from build123d import *

# Parameters (mm, degrees)
SKETCH2_R                = 107.15
BOSS_EXTRUDE2_DEPTH      = 70
BOSS_EXTRUDE2_DEPTH_BACK = 70
SKETCH10_R               = 19
CUT_EXTRUDE2_DEPTH       = 10
SKETCH18_R               = 22.5
BOSS_EXTRUDE6_DEPTH      = 32
BOSS_EXTRUDE6_DEPTH_BACK = 1
SKETCH56_R               = 30.95
BOSS_EXTRUDE7_DEPTH      = 5
BOSS_EXTRUDE7_DEPTH_BACK = 6
SKETCH20_R               = 104.1
CUT_EXTRUDE3_DEPTH       = 140
SKETCH51_R               = 2.5
CUT_EXTRUDE14_DEPTH      = 5
CUT_EXTRUDE14_DEPTH_BACK = 55
CUT_EXTRUDE15_DEPTH      = 5
SKETCH44_R               = 7.5
CUT_EXTRUDE10_DEPTH      = 10
FILLET3_R                = 1.5
SKETCH61_R               = 104.15
BOSS_EXTRUDE8_DEPTH      = 2
SKETCH62_R               = 102.15
CUT_EXTRUDE16_DEPTH      = 10
CHAMFER7_SIZE            = 1
CHAMFER7_SIZE2           = 0.700207538
SKETCH5_W                = 211.3
SKETCH5_H                = 3
BOSS_EXTRUDE3_DEPTH      = 24
SKETCH24_R               = 18.25
CUT_EXTRUDE6_DEPTH       = 50
SKETCH23_R               = 20.45
CUT_EXTRUDE5_DEPTH       = 7
CUT_EXTRUDE5_DEPTH_BACK  = 5
CHAMFER1_SIZE            = 0.5
FILLET4_R                = 0.6
CUT_EXTRUDE19_DEPTH      = 4


with BuildPart() as part:
    # Sketch2 → Boss-Extrude2 (new, two sides)
    with BuildSketch(Plane.XY) as boss_extrude2_sk:
        Circle(SKETCH2_R)
    extrude(amount=BOSS_EXTRUDE2_DEPTH)
    extrude(boss_extrude2_sk.sketch, amount=-BOSS_EXTRUDE2_DEPTH_BACK)

    # Sketch10 → Cut-Extrude2 (cut, symmetric)
    with BuildSketch(Plane(origin=(0, 51.109455148, -37.133192748), x_dir=(1, 0, 0), z_dir=(0, -0.8090169943749408, 0.5877852522924822))):
        with Locations((0, 95.341869558)):
            Circle(SKETCH10_R)
    extrude(amount=CUT_EXTRUDE2_DEPTH, both=True, mode=Mode.SUBTRACT)

    # Sketch18 → Boss-Extrude6 (add, two sides)
    with BuildSketch(Plane(origin=(0, 63.244710063, -45.949971532), x_dir=(1, 0, 0), z_dir=(0, -0.8090169943749408, 0.5877852522924822))) as boss_extrude6_sk:
        with Locations((0, 95.341869558)):
            Circle(SKETCH18_R)
    extrude(amount=BOSS_EXTRUDE6_DEPTH)
    extrude(boss_extrude6_sk.sketch, amount=-BOSS_EXTRUDE6_DEPTH_BACK)

    # Sketch56 → Boss-Extrude7 (add, two sides)
    with BuildSketch(Plane(origin=(0, -107.15, 0), x_dir=(1, 0, 0), z_dir=(0, 1, 0))) as boss_extrude7_sk:
        with Locations(Location((0, 1.5, 0), (0, 0, 270))):
            Circle(SKETCH56_R)
    extrude(amount=BOSS_EXTRUDE7_DEPTH)
    extrude(boss_extrude7_sk.sketch, amount=-BOSS_EXTRUDE7_DEPTH_BACK)

    # Sketch20 → Cut-Extrude3 (cut)
    with BuildSketch(Plane.XY.offset(70)):
        Circle(SKETCH20_R)
    extrude(amount=-CUT_EXTRUDE3_DEPTH, mode=Mode.SUBTRACT)

    # Sketch51 → Cut-Extrude14 (cut, two sides)
    with BuildSketch(Plane(origin=(0, -107.15, 0), x_dir=(1, 0, 0), z_dir=(0, 1, 0))) as cut_extrude14_sk:
        with Locations(Location((0, -24, 0), (0, 0, 90))):
            Circle(SKETCH51_R)
    extrude(amount=CUT_EXTRUDE14_DEPTH, mode=Mode.SUBTRACT)
    extrude(cut_extrude14_sk.sketch, amount=-CUT_EXTRUDE14_DEPTH_BACK, mode=Mode.SUBTRACT)

    # Sketch58 → Cut-Extrude15 (cut)
    with BuildSketch(Plane(origin=(0, -105.15, 0), x_dir=(1, 0, 0), z_dir=(0, 1, 0))):
        Polygon((0, -24), (1, -24), (1, -34.192827208), (-1, -34.192827208), (-1, -24), align=None)
    extrude(amount=CUT_EXTRUDE15_DEPTH, mode=Mode.SUBTRACT)

    # Sketch44 → Cut-Extrude10 (cut)
    with BuildSketch(Plane(origin=(0, -105.15, 0), x_dir=(1, 0, 0), z_dir=(0, 1, 0))):
        with Locations((0, -35.5)):
            Circle(SKETCH44_R)
    extrude(amount=CUT_EXTRUDE10_DEPTH, mode=Mode.SUBTRACT)

    # Fillet3
    fillet3_edges = [part.edges().sort_by_distance(p)[0] for p in [
        (0, -105.15, 26.5),
    ]]
    fillet(fillet3_edges, radius=FILLET3_R)

    # Sketch61 → Boss-Extrude8 (add)
    with BuildSketch(Plane.XY.offset(22)):
        Circle(SKETCH61_R)
    extrude(amount=-BOSS_EXTRUDE8_DEPTH)

    # Sketch62 → Cut-Extrude16 (cut)
    with BuildSketch(Plane.XY.offset(22)):
        Circle(SKETCH62_R)
    extrude(amount=-CUT_EXTRUDE16_DEPTH, mode=Mode.SUBTRACT)

    # Chamfer7
    chamfer7_edges = [part.edges().sort_by_distance(p)[0] for p in [
        (-102.15, 0, 20),
    ]]
    chamfer7_side = [part.faces().sort_by_distance(p)[0] for p in [
        (-102.15, 0, 21),
    ]]
    chamfer(chamfer7_edges, length=CHAMFER7_SIZE, length2=CHAMFER7_SIZE2, reference=chamfer7_side[0])

    # Sketch5 → Boss-Extrude3 (add)
    with BuildSketch(Plane.XY.offset(45)):
        Rectangle(SKETCH5_W, SKETCH5_H)
    extrude(amount=-BOSS_EXTRUDE3_DEPTH)

    # Sketch24 → Cut-Extrude6 (cut)
    with BuildSketch(Plane(origin=(0, 63.244710063, -45.949971532), x_dir=(1, 0, 0), z_dir=(0, -0.8090169943749408, 0.5877852522924822))):
        with Locations(Location((0, 95.341869558, 0), (0, 0, 244.88549582))):
            Circle(SKETCH24_R)
    extrude(amount=CUT_EXTRUDE6_DEPTH, mode=Mode.SUBTRACT)

    # Sketch23 → Cut-Extrude5 (cut, two sides)
    with BuildSketch(Plane(origin=(0, 63.244710063, -45.949971532), x_dir=(1, 0, 0), z_dir=(0, -0.8090169943749408, 0.5877852522924822))) as cut_extrude5_sk:
        with Locations(Location((0, 95.341869558, 0), (0, 0, 270))):
            Circle(SKETCH23_R)
    extrude(amount=CUT_EXTRUDE5_DEPTH, mode=Mode.SUBTRACT)
    extrude(cut_extrude5_sk.sketch, amount=-CUT_EXTRUDE5_DEPTH_BACK, mode=Mode.SUBTRACT)

    # Chamfer1
    chamfer1_edges = [part.edges().sort_by_distance(p)[0] for p in [
        (0, -113.15, -32.45),
    ]]
    chamfer(chamfer1_edges, length=CHAMFER1_SIZE)

    # Fillet4
    fillet4_edges = [part.edges().sort_by_distance(p)[0] for p in [
        (0, 132.114480319, 47.139833498),
    ]]
    fillet(fillet4_edges, radius=FILLET4_R)

    # Sketch67 → Cut-Extrude19 (cut)
    with BuildSketch(Plane(origin=(0, 57.581591103, -41.835474766), x_dir=(1, 0, 0), z_dir=(0, 0.8090169943749409, -0.5877852522924822))):
        Polygon((-7.872943576, -76.468097824), (7.872943576, -76.468097824), (7.872943576, -79.749667474), (-7.872943576, -79.48866005), align=None)
    extrude(amount=-CUT_EXTRUDE19_DEPTH, mode=Mode.SUBTRACT)


solid = part.part
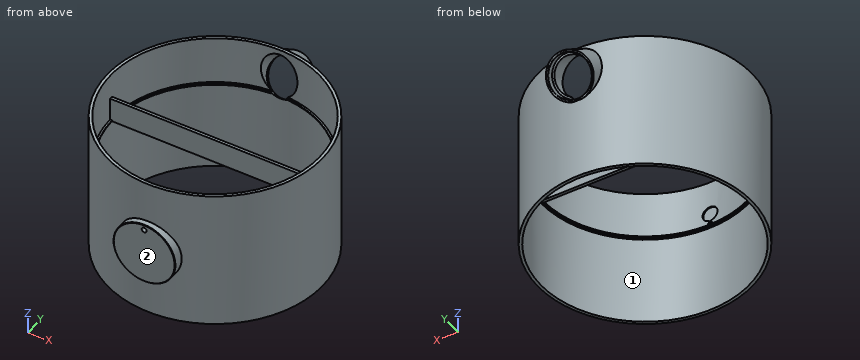
Design review of the part built by this model. Coordinates are the model's own, in mm. Face numbers are marked on the shaded views. Give positions to 0.01 mm unless a question says otherwise; leave off trailing zeros. Loops run counter-clockwise (first coordinate to the right, second up) from the corner with the lowest first, then second, coordinate; pieces in that order, holes last. Notation, with made-up numbers: (6, -14.5) - (39, -14.5) arc R10 ccw to (39, -10.5) - close; hole circle Ø6 at (-24, 63). An arc over 180 degrees is marked (long way). Use CSV: the item, a comma, the result in double quotes. Start each with the question number.
1. Draft analysis for pull direction Y (two halves, no side actions). For the marked faces 1 and 2, state which applies: released by +Y, released by -Y, zero draft, split by the parting line, or undercut.
2. Wall thickness on L1, parallel to Y at x = 89, z = 29.5; L2, parallel to Y at x = -3, z = -15; L3, parallel to Y at x = -95, z = 42: over which ranges is each line inside the solid? List them lowest first.
3. Add section B-B (x = 92). Count the separate pieces of the cut face and the enclosed holes in it, plus the area to 3 significant figures.
4. Insertion check: P1, Ø3, axis at x = -48.5, z = -37, coming from the +Y side; P2, Ø8, axis at x = 59, z = 44, coming from the -Y side; P3, Ø2.5, axis at x = 25, y = 0.5, coming from the -Z side. Each pin has a flat end and moves straight along its axis. Give the tip position at first contact, or say it passes through.
5. Add section A-A (z = -1.5). State the section outline as (x, y) points, plus the area to 3 significant figures.
Results found:
1,face 1,"undercut"
1,face 2,"released by -Y"
2,L1,"y = -59.67 to -54, -1.5 to 1.5, 54 to 59.67"
2,L2,"y = -113.15 to -104.06, 104.06 to 107.11"
2,L3,"y = -49.56 to -42.57, -1.5 to 1.5, 42.57 to 49.56"
3,separate pieces,"3"
3,enclosed holes,"0"
3,area,"1,830 mm²"
4,P1,"stops at y = 96.29"
4,P2,"stops at y = -91.96"
4,P3,"stops at z = 21"
5,outline,"(-30.95, -112.65) - (-30.45, -113.15) - (30.45, -113.15) - (30.95, -112.65) - (30.95, -102.58) arc R107.15 ccw (long way) to (-30.95, -102.58) - close; hole circle Ø208.2 at (0, 0)"
5,area,"2,490 mm²"
